Can you work these out from the model? Positions are in its coordinate system, mm. A direction names the side the tool comes from. Round coordinates to 2 decimals unless told otherwise and drop trailing zeros. Loops run counter-clockwise (first coordinate to the right, second up) from the corner with the lowest first, then second, coordinate; pieces in that order, holes last. Notation, with made-up numbers: (0.25, 36) -> (40.25, 36) arc R33 ccw to (40.25, 67) -> close; hole circle Ø2 at (45, -34). An arc over 180 degrees is marked (long way). Write each question's results on one line, items separated by ' | '.
from build123d import *

# Parameters (mm, degrees)
SKETCH_1_R             = 13.45
SKETCH_1_R_2           = 10.5
EXTRUDE_1_DEPTH        = 60
EXTRUDE_1_2_DEPTH      = 47
EXTRUDE_1_2_DEPTH_BACK = 5
SKETCH_2_W             = 14
SKETCH_2_H             = 27


with BuildPart() as part:
    # 草圖1 → Extrude 1 (new body)
    with BuildSketch(Plane(origin=(0, 0, 0), x_dir=(1, 0, 0), z_dir=(0, 1, 0))):
        Circle(SKETCH_1_R)
        Circle(SKETCH_1_R_2, mode=Mode.SUBTRACT)
    extrude(amount=EXTRUDE_1_DEPTH)

    # 草圖2 → Extrude 1 2 (add, two sides: drawn at the far end of the back side and taken through both)
    with BuildSketch(Plane(origin=(10, 0, 0), x_dir=(0, 0, -1), z_dir=(1, 0, 0)).offset(-EXTRUDE_1_2_DEPTH_BACK)):
        with Locations((0, 37.071329062)):
            Rectangle(SKETCH_2_W, SKETCH_2_H)
    extrude(amount=EXTRUDE_1_2_DEPTH + EXTRUDE_1_2_DEPTH_BACK)


solid = part.part
1. Will these pins go through, and if not, where does the flat tip stop? pin 1 (1.4 mm diameter, centred on x = 6.5, y = 31, fed in from -Z); pin 2 (3 mm diameter, centred on y = 38.5, z = -5, fed in from -X); pin 3 (13.5 mm diameter, centred on x = 31, y = 30.5, fed in from -Z); pin 4 (8 mm diameter, centred on x = -1.5, z = 1.5, fed in from +Y).
Final values:
pin 1: z = -12.14 | pin 2: x = -12.99 | pin 3: z = -7 | pin 4: through
2. Please list where these lines run through material, in increasing order: line 1 (Z direction, x = 0, y = 48); line 2 (Y direction, x = 14, z = 3). Write a range as from..to.
Final values:
line 1: -13.45..-10.5, 10.5..13.45 | line 2: 23.57..50.57
3. We'd pull the mould along X, two halves only. Please class faces 5 (the face through (57, 37, 0)), 6 (the face through (5, 37, 0)), 7 (the face through (-13.437, 29.58, -0.591)): pulls with the +X half, pulls with the -X half, needs draft (parallel to the pull), parting line crosses it, or undercut.
Final values:
face 5: pulls with the +X half | face 6: undercut | face 7: parting line crosses it
4. If we section it at B-B (z = 0): List the corners of the cut face in (x, y) for me, then the cut area to 3 significant figures.
Final values:
outline: (-13.45, 0) -> (-10.5, 0) -> (-10.5, 60) -> (-13.45, 60) -> close; (5, 23.57) -> (10.5, 23.57) -> (10.5, 0) -> (13.45, 0) -> (13.45, 23.57) -> (57, 23.57) -> (57, 50.57) -> (13.45, 50.57) -> (13.45, 60) -> (10.5, 60) -> (10.5, 50.57) -> (5, 50.57) -> close | area: 1,680 mm2
5. If we section it at D-D (z = -4.5): List the corners of the cut face in (x, y) for me, then the cut area to 3 significant figures.
Final values:
outline: (-12.67, 0) -> (-9.49, 0) -> (-9.49, 60) -> (-12.67, 60) -> close; (5, 23.57) -> (9.49, 23.57) -> (9.49, 0) -> (12.67, 0) -> (12.67, 23.57) -> (57, 23.57) -> (57, 50.57) -> (12.67, 50.57) -> (12.67, 60) -> (9.49, 60) -> (9.49, 50.57) -> (5, 50.57) -> close | area: 1,700 mm2
6. If we section it at C-C (y = 13.5): List the corners of the cut face in (x, z) for me, then the cut area to 3 significant figures.
Final values:
outline: circle Ø26.9 at (0, 0); hole circle Ø21 at (0, 0) | area: 222 mm2
7. If we section it at A-A (x = 0): List the corners of the cut face in (y, z) for me, then the cut area to 3 significant figures.
Final values:
outline: (0, -13.45) -> (60, -13.45) -> (60, -10.5) -> (0, -10.5) -> close; (0, 10.5) -> (60, 10.5) -> (60, 13.45) -> (0, 13.45) -> close | area: 354 mm2
8. On a 3-axis mill with a long thin cutter (end or side, diameter ignored), from which of +Z, -Z, +X, -X, +Y, -Y can I reach the whole of each face in a straight line? I mean faces 1 (the face through (34, 37, -7)), 2 (the face through (7, 50.571, 0)), 3 (the face through (34, 37, 7)), 4 (the face through (7, 23.571, 0)). Say none if no direction works.
Final values:
face 1: -Z, +X, +Y, -Y | face 2: +Y | face 3: +Z, +X, +Y, -Y | face 4: -Y
